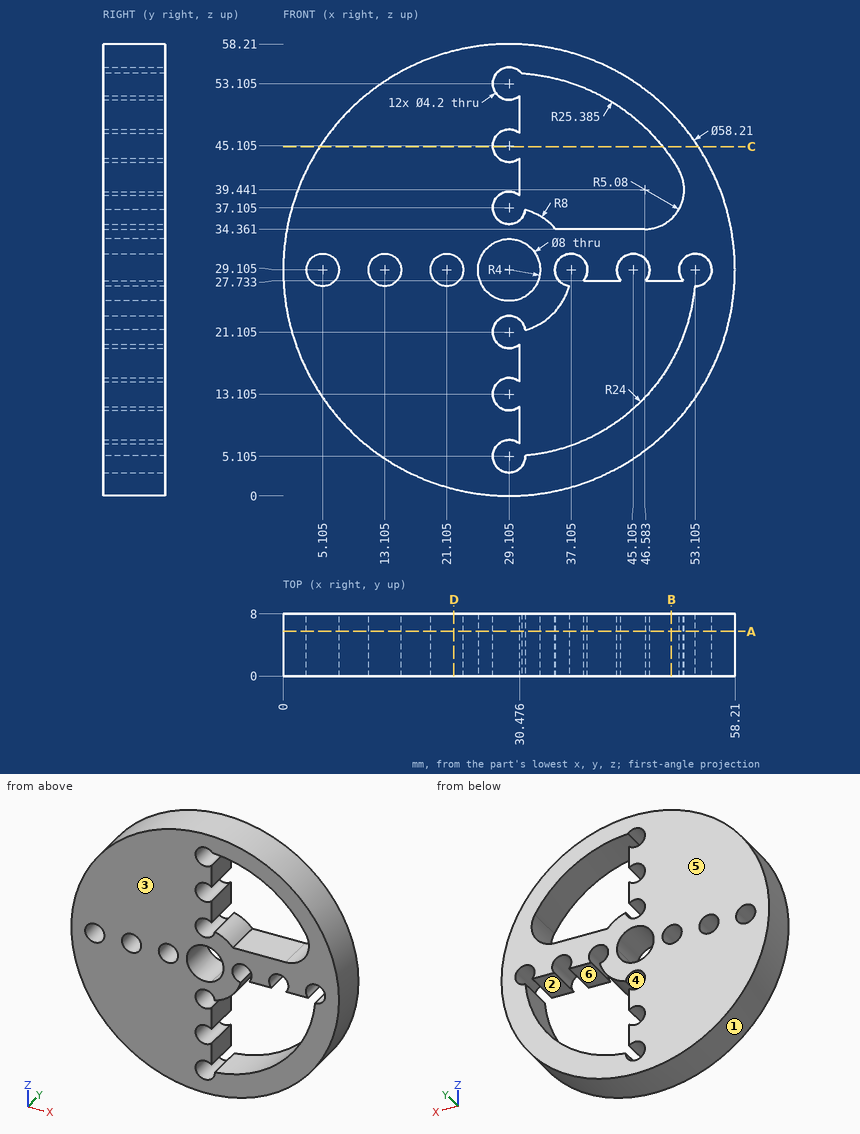
Study the drawing (mm; zero at the part's minimum x, y, z) and answer. A direction names the side the tool comes from. Round coordinates to 2 decimals unless told otherwise and drop trailing zeros. Write each loop counter-clockwise with the first axis right and the second up, starting at its lowest first coordinate (ties: lowest second). Pieces come first, ordered by that corner, then holes. Notation, with made-up numbers: (81.25, 81.25) -> (137.25, 81.25) arc R20 ccw to (137.25, 98.25) -> close; hole circle Ø6 at (11, -38.75). An arc over 180 degrees is marked (long way). Answer as CSV lines item,"result". Start each with the question number.
(1) The part is cut by section C-C, the plane z = 45. Give the vertices of the cut face in (x, y).
(2) The part is cut by section A-A, the plane y = 5.75. Give the vertices of the cut face in (x, z) (1 decimal).
(3) The part is cut by section B-B, the plane x = 50. Give the vertices of the cut face in (y, z) (1 decimal), then the cut area to 3 significant figures.
(4) The mould has two halves that part along X. Classify the marked faces 1, 2, 3 and 4: +X half, -X half, draft (parallel to the pull), parting line (faces both ways), or undercut.
(5) Each of these flat-tipped pins is pushed along its axis until it touches: pin 1 (1.5 mm diameter, centred on y = 2.5, z = 18.5, fed in from +X); pin 2 (4 mm diameter, centred on x = 30.5, y = 1.5, fed in from -Z); pin 3 (2.5 mm diameter, centred on x = 40.5, y = 3, fed in from -Z) (1 decimal). Where does it stop, or does it pass through?
(6) A tool of negligible diameter and unlimited length cuts with its end or side. For the marked faces 5 and 6, from which of +Z, -Z, +X, -X, +Y, -Y can it reach the whole face along a straight path? Write none if from no direction.
(7) Find the intervals of material crossed by probe 1 along Z at (x, y) = (38, 1.25) (1 decimal); probe 2 along Z at (x, y) = (39.5, 5.5) (1 decimal); probe 3 along X at (y, z) = (7.75, 16.5) (1 decimal), in increasing order.
(8) The part is cut by section D-D, the plane x = 22. Give the vertices of the cut face in (y, z) (1 decimal).
Output values:
1,outline,"(4.72, 0) -> (27.01, 0) -> (27.01, 8) -> (4.72, 8) -> close; (48.9, 0) -> (53.49, 0) -> (53.49, 8) -> (48.9, 8) -> close"
2,outline,"circle Ø58.2 at (29.1, 29.1); hole circle Ø4.2 at (5.1, 29.1); hole circle Ø4.2 at (13.1, 29.1); hole circle Ø4.2 at (21.1, 29.1); hole circle Ø8 at (29.1, 29.1); hole (30.5, 6.7) arc R2.1 ccw (long way) to (31.2, 5.2) arc R24 ccw to (53, 27) arc R2.1 ccw (long way) to (51.5, 27.7) -> (46.7, 27.7) arc R2.1 ccw (long way) to (43.5, 27.7) -> (38.7, 27.7) arc R2.1 ccw (long way) to (36.8, 27) arc R8 cw to (31.2, 21.4) arc R2.1 ccw (long way) to (30.5, 19.5) -> (30.5, 14.7) arc R2.1 ccw (long way) to (30.5, 11.5) -> close; hole (30.5, 38.7) arc R2.1 ccw (long way) to (31.2, 36.8) arc R8 cw to (35.1, 34.4) -> (46.6, 34.4) arc R5.1 ccw to (51, 42) arc R25.4 ccw to (30.7, 54.4) arc R2.1 ccw (long way) to (30.5, 51.5) -> (30.5, 46.7) arc R2.1 ccw (long way) to (30.5, 43.5) -> close"
3,outline,"(0, 8.8) -> (8, 8.8) -> (8, 17.3) -> (0, 17.3) -> close; (0, 27.7) -> (8, 27.7) -> (8, 35.7) -> (0, 35.7) -> close; (0, 43.5) -> (8, 43.5) -> (8, 49.4) -> (0, 49.4) -> close"
3,area,"178 mm²"
4,face 1,"parting line"
4,face 2,"undercut"
4,face 3,"draft"
4,face 4,"undercut"
5,pin 1,"stops at x = 56.49"
5,pin 2,"stops at z = 0"
5,pin 3,"stops at z = 1.8"
6,face 5,"+Z, -Z, +X, -X, +Y"
6,face 6,"+Y, -Y"
7,probe 1,"z = 1.4 to 6.8, 31 to 34.4, 52.9 to 56.8"
7,probe 2,"z = 1.9 to 7.5, 27.7 to 34.4, 52.3 to 56.3"
7,probe 3,"x = 2.9 to 30.5, 49.5 to 55.3"
8,outline,"(0, 0.9) -> (8, 0.9) -> (8, 27.2) -> (0, 27.2) -> close; (0, 31) -> (8, 31) -> (8, 57.3) -> (0, 57.3) -> close"
